Here's how the part is built. I have some questions about the finished solid (model axes, mm). A direction names the side the tool comes from. Round coordinates to 2 decimals unless told otherwise and drop trailing zeros. Write each loop counter-clockwise with the first axis right and the second up, starting at its lowest first coordinate (ties: lowest second). Pieces come first, ordered by that corner, then holes. Notation, with made-up numbers: M 60.25,-25.75 L 118.25,-25.75 A26 ccw 118.25,-5.75 Z; hole C 61.5,-34 d6. An arc over 180 degrees is marked long. Use a Markdown table: item, result. Add a question column.
```python
from build123d import *

# Parameters (mm, degrees)
ESQUISSE1_W             = 210
ESQUISSE1_H             = 44
BOSS_EXTRU_1_DEPTH      = 8
ESQUISSE2_R             = 2.75
ENL_V_MAT_EXTRU_1_DEPTH = 9
CHANFREIN1_SIZE         = 2.5
ENL_V_MAT_EXTRU_2_DEPTH = 9
ESQUISSE4_R             = 1.65
ENL_V_MAT_EXTRU_3_DEPTH = 9
ESQUISSE5_R             = 1.65
ENL_V_MAT_EXTRU_4_DEPTH = 8
ESQUISSE6_R             = 1.65
ENL_V_MAT_EXTRU_5_DEPTH = 8


with BuildPart() as part:
    # Esquisse1 → Boss.-Extru.1 (new body)
    with BuildSketch(Plane.XY):
        with Locations((31.855664279, -10.840611814)):
            Rectangle(ESQUISSE1_W, ESQUISSE1_H)
    extrude(amount=BOSS_EXTRU_1_DEPTH)

    # Esquisse2 → Enlèv. mat.-Extru.1 (cut, through all)
    with BuildSketch(Plane.XY.offset(8)):
        with Locations((-67.144335721, 5.159388186)):
            Circle(ESQUISSE2_R)
        with Locations((-67.144335721, -26.840611814)):
            Circle(ESQUISSE2_R)
        with Locations((-50.144335721, 5.159388186)):
            Circle(ESQUISSE2_R)
        with Locations((-50.144335721, -26.840611814)):
            Circle(ESQUISSE2_R)
        with Locations((130.855664279, 5.159388186)):
            Circle(ESQUISSE2_R)
        with Locations((130.855664279, -26.840611814)):
            Circle(ESQUISSE2_R)
        with Locations((113.855664279, 5.159388186)):
            Circle(ESQUISSE2_R)
        with Locations((113.855664279, -26.840611814)):
            Circle(ESQUISSE2_R)
    extrude(amount=-ENL_V_MAT_EXTRU_1_DEPTH, mode=Mode.SUBTRACT)

    # Chanfrein1
    chanfrein1_edges = [part.edges().sort_by_distance(p)[0] for p in [
        (-69.894335721, 5.159388186, 8),
        (-69.894335721, -26.840611814, 8),
        (-52.894335721, 5.159388186, 8),
        (-52.894335721, -26.840611814, 8),
        (128.105664279, 5.159388186, 8),
        (128.105664279, -26.840611814, 8),
        (111.105664279, 5.159388186, 8),
        (111.105664279, -26.840611814, 8),
    ]]
    chamfer(chanfrein1_edges, length=CHANFREIN1_SIZE)

    # Esquisse3 → Enlèv. mat.-Extru.2 (cut, through all)
    with BuildSketch(Plane.XY.offset(8)):
        with BuildLine():
            Line((-8.144335721, -4.840611814), (71.855664279, -4.840611814))
            ThreePointArc((71.855664279, -4.840611814), (77.855664279, -10.840611814), (71.855664279, -16.840611814))
            Line((71.855664279, -16.840611814), (-8.144335721, -16.840611814))
            ThreePointArc((-8.144335721, -16.840611814), (-14.144335721, -10.840611814), (-8.144335721, -4.840611814))
        make_face()
    extrude(amount=-ENL_V_MAT_EXTRU_2_DEPTH, mode=Mode.SUBTRACT)

    # Esquisse4 → Enlèv. mat.-Extru.3 (cut, through all)
    with BuildSketch(Plane.XY.offset(8)):
        with Locations((-58.644335721, -17.840611814)):
            Circle(ESQUISSE4_R)
        with Locations((-58.644335721, -3.840611814)):
            Circle(ESQUISSE4_R)
        with Locations((-23.644335721, -3.840611814)):
            Circle(ESQUISSE4_R)
        with Locations((-23.644335721, -17.840611814)):
            Circle(ESQUISSE4_R)
        with Locations((87.355664279, -3.840611814)):
            Circle(ESQUISSE4_R)
        with Locations((87.355664279, -17.840611814)):
            Circle(ESQUISSE4_R)
        with Locations((122.355664279, -3.840611814)):
            Circle(ESQUISSE4_R)
        with Locations((122.355664279, -17.840611814)):
            Circle(ESQUISSE4_R)
        with Locations((31.855664279, -0.840611814)):
            Circle(ESQUISSE4_R)
        with Locations((31.855664279, -20.840611814)):
            Circle(ESQUISSE4_R)
    extrude(amount=-ENL_V_MAT_EXTRU_3_DEPTH, mode=Mode.SUBTRACT)

    # Esquisse5 → Enlèv. mat.-Extru.4 (cut)
    with BuildSketch(Plane(origin=(0, 11.159388186, 0), x_dir=(1, 0, 0), z_dir=(0, 1, 0))):
        with Locations(Location((-58.644335721, -4, 0), (0, 0, 270))):  # turned: the seam where the file's is
            Circle(ESQUISSE5_R)
        with Locations(Location((-23.644335721, -4, 0), (0, 0, 270))):  # turned: the seam where the file's is
            Circle(ESQUISSE5_R)
        with Locations(Location((87.355664279, -4, 0), (0, 0, 270))):  # turned: the seam where the file's is
            Circle(ESQUISSE5_R)
        with Locations(Location((122.355664279, -4, 0), (0, 0, 270))):  # turned: the seam where the file's is
            Circle(ESQUISSE5_R)
        with Locations(Location((31.855664279, -4, 0), (0, 0, 270))):  # turned: the seam where the file's is
            Circle(ESQUISSE5_R)
    extrude(amount=-ENL_V_MAT_EXTRU_4_DEPTH, mode=Mode.SUBTRACT)

    # Esquisse6 → Enlèv. mat.-Extru.5 (cut)
    with BuildSketch(Plane.XZ.offset(32.840611814)):
        with Locations(Location((-58.644335721, 4, 0), (0, 0, 90))):  # turned: the seam where the file's is
            Circle(ESQUISSE6_R)
        with Locations(Location((-23.644335721, 4, 0), (0, 0, 90))):  # turned: the seam where the file's is
            Circle(ESQUISSE6_R)
        with Locations(Location((87.355664279, 4, 0), (0, 0, 90))):  # turned: the seam where the file's is
            Circle(ESQUISSE6_R)
        with Locations(Location((122.355664279, 4, 0), (0, 0, 90))):  # turned: the seam where the file's is
            Circle(ESQUISSE6_R)
        with Locations(Location((31.855664279, 4, 0), (0, 0, 90))):  # turned: the seam where the file's is
            Circle(ESQUISSE6_R)
    extrude(amount=-ENL_V_MAT_EXTRU_5_DEPTH, mode=Mode.SUBTRACT)


solid = part.part
```
Item 1: Imagine slicing it at B-B on z = 4. Count the separate pieces of the cut face and the enclosed holes in it, plus the area to 3 significant figures.
Item 2: For pin 1 Ø4.5 at (x, y) = (-50.14, 5.16) entering from -Z; pin 2 Ø2.5 at (x, z) = (122.5, 4) entering from -Y; pin 3 Ø2.5 at (x, z) = (122.36, 4) entering from +Y; pin 4 Ø9 at (x, y) = (130.86, 5.16) entering from +Z, each with a flat end and sliding along its axis, tell me the tip position at first contact or that it passes through.
Item 3: I need wall thicknesses on probe 1 along X at (y, z) = (-30, 4); probe 2 along Y at (x, z) = (87.5, 3.5); probe 3 along Y at (x, z) = (38, 5.75). Which ranges of each line are inside material? Lowest first, please. Write a range as from..to.
Item 4: On a 3-axis mill with a long thin cutter (end or side, diameter ignored), from which of +Z, -Z, +X, -X, +Y, -Y can I reach the whole of each face in a straight line? I mean faces 1 (the face through (116.396, 4.106, 2.788)), 2 (the face through (-60.11, 7.22, 4.76)), 3 (the face through (88.966, -28.897, 3.642)). Say none if no direction works.
Item 5: If we mould it in two halves opening along Z, with no side actions, what happens to faces 4 (the face through (127.99, 5.29, 5.62)), 5 (the face through (-25.255, 7.215, 3.642)), 6 (the face through (-52.89, -26.72, 2.79))? For each: +Z half, -Z half, draft (parallel to the pull), parting line (faces both ways), or undercut.
Item 6: Imagine slicing it at A-A on x = 53. List the corners of the cut face in (y, z) for me.
The answers:
| question | item | result |
|---|---|---|
| 1 | separate pieces | 1 |
| 1 | enclosed holes | 19 |
| 1 | area | 7,630 mm² |
| 2 | pin 1 | through |
| 2 | pin 2 | y = -24.84 |
| 2 | pin 3 | y = 3.16 |
| 2 | pin 4 | z = 7.25 |
| 3 | probe 1 | -73.14..-60.29, -56.99..-25.29, -21.99..30.21, 33.51..85.71, 89.01..120.71, 124.01..136.86 |
| 3 | probe 2 | -24.84..-19.48, -16.2..-5.48, -2.2..3.16 |
| 3 | probe 3 | -32.84..-16.84, -4.84..11.16 |
| 4 | face 1 | +Z, -Z |
| 4 | face 2 | +Y |
| 4 | face 3 | -Y |
| 5 | face 4 | +Z half |
| 5 | face 5 | undercut |
| 5 | face 6 | draft |
| 6 | outline | M -32.84,0 L -16.84,0 L -16.84,8 L -32.84,8 Z; M -4.84,0 L 11.16,0 L 11.16,8 L -4.84,8 Z |
